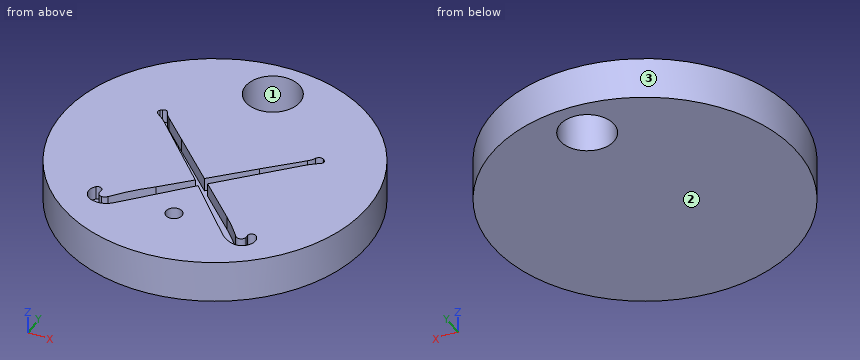
```python
from build123d import *

# Parameters (mm, degrees)
F0_R     = 11.27
F1_DEPTH = 3.14
F2_R     = 0.5890094212
F3_DEPTH = 1
F4_D     = 4


with BuildPart() as f1:
    # F0 (on Top) → F1 (new body)
    with BuildSketch(Plane.XY):
        Circle(F0_R)
    extrude(amount=F1_DEPTH)

    # F2 (on face) → F3 (cut)
    with BuildSketch(Plane.XY.offset(3.14)):
        with BuildLine():
            Line((-61.7312958373, 21.3926987009), (-58.0294454006, 25.2554991458))
            Line((-58.0294454006, 25.2554991458), (-54.1867637143, 21.2518673281))
            ThreePointArc((-54.1867637143, 21.2518673281), (-53.7373686171, 20.8806710534), (-53.2149149093, 20.6222435956))
            ThreePointArc((-53.2149149093, 20.6222435956), (-52.303276006, 20.7518245546), (-51.8888391992, 21.5740890181))
            ThreePointArc((-51.8888391992, 21.5740890181), (-51.9310478545, 21.7908044873), (-52.0434124717, 21.9808606841))
            ThreePointArc((-52.0434124717, 21.9808606841), (-52.3852964474, 22.1363147434), (-52.6291636905, 21.8506936919))
            Line((-52.6291636905, 21.8506936919), (-52.6291636905, 21.6066308894))
            ThreePointArc((-52.6291636905, 21.6066308894), (-52.9032514772, 21.281470401), (-53.2962690946, 21.4439222723))
            ThreePointArc((-53.2962690946, 21.4439222723), (-53.9894142385, 22.2523776329), (-54.7349330148, 23.012806469))
            Line((-54.7349330148, 23.012806469), (-57.5646452943, 25.7127153939))
            Line((-57.5646452943, 25.7127153939), (-54.5263338413, 28.7611883431))
            Line((-54.5263338413, 28.7611883431), (-52.9285208167, 30.355923602))
            ThreePointArc((-52.9285208167, 30.355923602), (-52.4977416389, 30.7470238341), (-52.0319618331, 31.0957060162))
            ThreePointArc((-52.0319618331, 31.0957060162), (-51.882280216, 31.3348975172), (-52.0319618331, 31.5740890181))
            ThreePointArc((-52.0319618331, 31.5740890181), (-52.3412808676, 31.6540069056), (-52.5764442328, 31.4377586097))
            ThreePointArc((-52.5764442328, 31.4377586097), (-52.720584525, 31.1912058371), (-52.9093169978, 30.9768585785))
            Line((-52.9093169978, 30.9768585785), (-55.3087755022, 28.7307036543))
            Line((-55.3087755022, 28.7307036543), (-58.0172568554, 26.1346496445))
            Line((-58.0172568554, 26.1346496445), (-61.3351414896, 29.3003376902))
            Line((-61.3351414896, 29.3003376902), (-63.1147513893, 30.9945066363))
            ThreePointArc((-63.1147513893, 30.9945066363), (-63.2699523014, 31.1530129011), (-63.4136438076, 31.3220226943))
            ThreePointArc((-63.4136438076, 31.3220226943), (-63.4713878606, 31.4628315528), (-63.5582546894, 31.5877942045))
            ThreePointArc((-63.5582546894, 31.5877942045), (-63.7382128733, 31.6951710938), (-63.9334617012, 31.6190617019))
            Line((-63.9334617012, 31.6190617019), (-64.0585307051, 31.5174429514))
            ThreePointArc((-64.0585307051, 31.5174429514), (-64.1366278816, 31.3000099116), (-64.0038129543, 31.1109689349))
            Line((-64.0038129543, 31.1109689349), (-63.8474769458, 30.9898083066))
            ThreePointArc((-63.8474769458, 30.9898083066), (-63.4886568855, 30.7229218485), (-63.1577918353, 30.4220754827))
            Line((-63.1577918353, 30.4220754827), (-62.9491744453, 30.2127408469))
            Line((-62.9491744453, 30.2127408469), (-58.4760000401, 25.7241872536))
            Line((-58.4760000401, 25.7241872536), (-60.4066995048, 23.874780467))
            ThreePointArc((-60.4066995048, 23.874780467), (-61.6253233945, 22.738509753), (-62.7133773323, 21.4766484497))
            ThreePointArc((-62.7133773323, 21.4766484497), (-62.8851672484, 21.3450641448), (-63.089355572, 21.2734168623))
            ThreePointArc((-63.089355572, 21.2734168623), (-63.3925338367, 21.4837956535), (-63.404364434, 21.8526266894))
            ThreePointArc((-63.404364434, 21.8526266894), (-63.5864183589, 22.1403709739), (-63.9226048834, 22.0863429656))
            ThreePointArc((-63.9226048834, 22.0863429656), (-64.0836440025, 21.1552024698), (-63.3027486402, 20.6230759303))
            ThreePointArc((-63.3027486402, 20.6230759303), (-62.6464252626, 20.6724715017), (-62.0935210892, 21.0295391052))
            Line((-62.0935210892, 21.0295391052), (-61.7312958373, 21.3926987009))
        make_face()
        with BuildLine():
            Line((-3.4236896342, -6.8191600484), (0.2781608025, -2.9563596035))
            Line((0.2781608025, -2.9563596035), (4.1208424888, -6.9599914212))
            ThreePointArc((4.1208424888, -6.9599914212), (4.570237586, -7.3311876959), (5.0926912938, -7.5896151537))
            ThreePointArc((5.0926912938, -7.5896151537), (6.004330197, -7.4600341947), (6.4187670038, -6.6377697312))
            ThreePointArc((6.4187670038, -6.6377697312), (6.3765583485, -6.421054262), (6.2641937313, -6.2309980652))
            ThreePointArc((6.2641937313, -6.2309980652), (5.9223097557, -6.0755440059), (5.6784425126, -6.3611650574))
            Line((5.6784425126, -6.3611650574), (5.6784425126, -6.6052278599))
            ThreePointArc((5.6784425126, -6.6052278599), (5.4043547258, -6.9303883483), (5.0113371085, -6.767936477))
            ThreePointArc((5.0113371085, -6.767936477), (4.3181919645, -5.9594811164), (3.5726731882, -5.1990522803))
            Line((3.5726731882, -5.1990522803), (0.7429609088, -2.4991433554))
            Line((0.7429609088, -2.4991433554), (3.7812723618, 0.5493295938))
            Line((3.7812723618, 0.5493295938), (5.3790853864, 2.1440648527))
            ThreePointArc((5.3790853864, 2.1440648527), (5.8098645642, 2.5351650848), (6.2756443699, 2.8838472669))
            ThreePointArc((6.2756443699, 2.8838472669), (6.4253259871, 3.1230387679), (6.2756443699, 3.3622302688))
            ThreePointArc((6.2756443699, 3.3622302688), (5.9663253355, 3.4421481563), (5.7311619703, 3.2258998604))
            ThreePointArc((5.7311619703, 3.2258998604), (5.587021678, 2.9793470878), (5.3982892053, 2.7649998292))
            Line((5.3982892053, 2.7649998292), (2.9988307009, 0.518844905))
            Line((2.9988307009, 0.518844905), (0.2903493477, -2.0772091048))
            Line((0.2903493477, -2.0772091048), (-3.0275352865, 1.0884789409))
            Line((-3.0275352865, 1.0884789409), (-4.8071451862, 2.782647887))
            ThreePointArc((-4.8071451862, 2.782647887), (-4.9623460984, 2.9411541518), (-5.1060376045, 3.110163945))
            ThreePointArc((-5.1060376045, 3.110163945), (-5.1637816575, 3.2509728035), (-5.2506484863, 3.3759354552))
            ThreePointArc((-5.2506484863, 3.3759354552), (-5.4306066702, 3.4833123445), (-5.6258554981, 3.4072029526))
            Line((-5.6258554981, 3.4072029526), (-5.7509245021, 3.3055842021))
            ThreePointArc((-5.7509245021, 3.3055842021), (-5.8290216786, 3.0881511623), (-5.6962067512, 2.8991101857))
            Line((-5.6962067512, 2.8991101857), (-5.5398707427, 2.7779495573))
            ThreePointArc((-5.5398707427, 2.7779495573), (-5.1810506824, 2.5110630992), (-4.8501856322, 2.2102167334))
            Line((-4.8501856322, 2.2102167334), (-4.6415682422, 2.0008820976))
            Line((-4.6415682422, 2.0008820976), (-0.168393837, -2.4876714957))
            Line((-0.168393837, -2.4876714957), (-2.0990933017, -4.3370782823))
            ThreePointArc((-2.0990933017, -4.3370782823), (-3.3177171915, -5.4733489963), (-4.4057711293, -6.7352102996))
            ThreePointArc((-4.4057711293, -6.7352102996), (-4.5775610453, -6.8667946045), (-4.7817493689, -6.938441887))
            ThreePointArc((-4.7817493689, -6.938441887), (-5.0849276337, -6.7280630958), (-5.0967582309, -6.3592320599))
            ThreePointArc((-5.0967582309, -6.3592320599), (-5.2788121559, -6.0714877754), (-5.6149986803, -6.1255157836))
            ThreePointArc((-5.6149986803, -6.1255157836), (-5.7760377995, -7.0566562795), (-4.9951424372, -7.588782819))
            ThreePointArc((-4.9951424372, -7.588782819), (-4.3388190596, -7.5393872476), (-3.7859148861, -7.1823196441))
            Line((-3.7859148861, -7.1823196441), (-3.4236896342, -6.8191600484))
        make_face()
        with Locations((0.2781608025, -6.4016040415)):
            Circle(F2_R)
    extrude(amount=-F3_DEPTH, mode=Mode.SUBTRACT)

    # F4 (through all)
    with Locations(Plane(origin=(0, 0, 0), x_dir=(1, 0, 0), z_dir=(0, 0, -1))):
        with Locations((0, -8.27)):
            Hole(F4_D / 2)


solid = f1.part
```
Could you check a few things on this model? Use its own coordinates, in mm. Face numbers are marked on the shaded views. Coordinates: 2 decimals unless noted, no trailing zeros. Write each loop counter-clockwise with the first axis right and the second up, starting at its lowest first coordinate (ties: lowest second). Pieces come first, ordered by that corner, then holes. Notation, with made-up numbers: (-14, 73) -> (31, 73) arc R30 ccw to (31, 109) -> close; hole circle Ø6 at (73.5, -33.75). An arc over 180 degrees is marked (long way). Write item = value, one per line. Start each with the question number.
(1) I want a section at A-A (y = 8.27). Please give me the cut outline in (x, z).
(2) I want a section at B-B (z = 0.9). Please give me the cut outline in (x, y).
(3) I want a section at C-C (y = 0). Please give me the cut outline in (x, z).
(4) I need wall thicknesses on line 1 (Y direction, x = -3.75, z = 2.75); line 2 (Y direction, x = 0, z = 1.7); line 3 (X direction, y = 8.75, z = 2.1). Which ranges of each line are inside material? Lowest first, please. Write a range as [from, to].
(5) We'd pull the mould along X, two halves only. Please class the marked faces 1, 2 and 3: released by +X, released by -X, zero draft, split by the parting line, or undercut.
(6) I want a section at D-D (x = 9.25). Please give me the cut outline in (y, z), plus the area to 3 significant figures.
(7) Will this pin go through, and if not, where does the flat tip stop? pin 1 (3 mm diameter, centred on x = -1, y = -7.5, fed in from -Z).
Result set:
q1.outline = (-7.66, 0) -> (-2, 0) -> (-2, 3.14) -> (-7.66, 3.14) -> close; (2, 0) -> (7.66, 0) -> (7.66, 3.14) -> (2, 3.14) -> close
q2.outline = circle Ø22.54 at (0, 0); hole circle Ø4 at (0, 8.27)
q3.outline = (-11.27, 0) -> (11.27, 0) -> (11.27, 3.14) -> (3.23, 3.14) -> (3.23, 2.14) -> (2.46, 2.14) -> (2.46, 3.14) -> (-1.89, 3.14) -> (-1.89, 2.14) -> (-2.65, 2.14) -> (-2.65, 3.14) -> (-11.27, 3.14) -> close
q4.line_1 = [-10.63, -7.15], [-5.94, 1.11], [1.78, 10.63]
q4.line_2 = [-11.27, 6.27], [10.27, 11.27]
q4.line_3 = [-7.1, -1.94], [1.94, 7.1]
q5.face_1 = undercut
q5.face_2 = zero draft
q5.face_3 = split by the parting line
q6.outline = (-6.44, 0) -> (6.44, 0) -> (6.44, 3.14) -> (-6.44, 3.14) -> close
q6.area = 40.4 mm2
q7.pin_1 = 0
